Here's the drawing with two shaded views (mm, measured from the low corner). I have some questions. Coordinates: 2 decimals unless noted, no trailing zeros. Write each loop counter-clockwise with the first axis right and the second up, starting at its lowest first coordinate (ties: lowest second). Pieces come first, ordered by that corner, then holes.
Item 1: I want a section at B-B on z = 188.5. Please give me the cut outline in (x, y), then the cut area to 3 significant figures.
Item 2: For P1, Ø8, axis at x = 82.5, y = 184, coming from the -Z side, with a flat end and sliding along its axis, tell me the tip position at first contact or that it passes through.
Item 3: Thinking about a two-plate mould opening in Y: for the marked faces 1 and 2, which applies, +Y half, -Y half, draft (parallel to the pull), parting line (faces both ways), or undercut?
Item 4: I want a section at D-D on x = 172.5. Please give me the cut outline in (y, z).
Item 5: I want a section at A-A on y = 425. Please give me the cut outline in (x, z).
Item 6: If I drill on probe 1 along X at (y, z) = (24, 268); probe 2 along Z at (x, y) = (128, 170.5); probe 3 along X at (y, z) = (428.5, 295.5), over which ranges is the centre line in solid material (lowest first)?
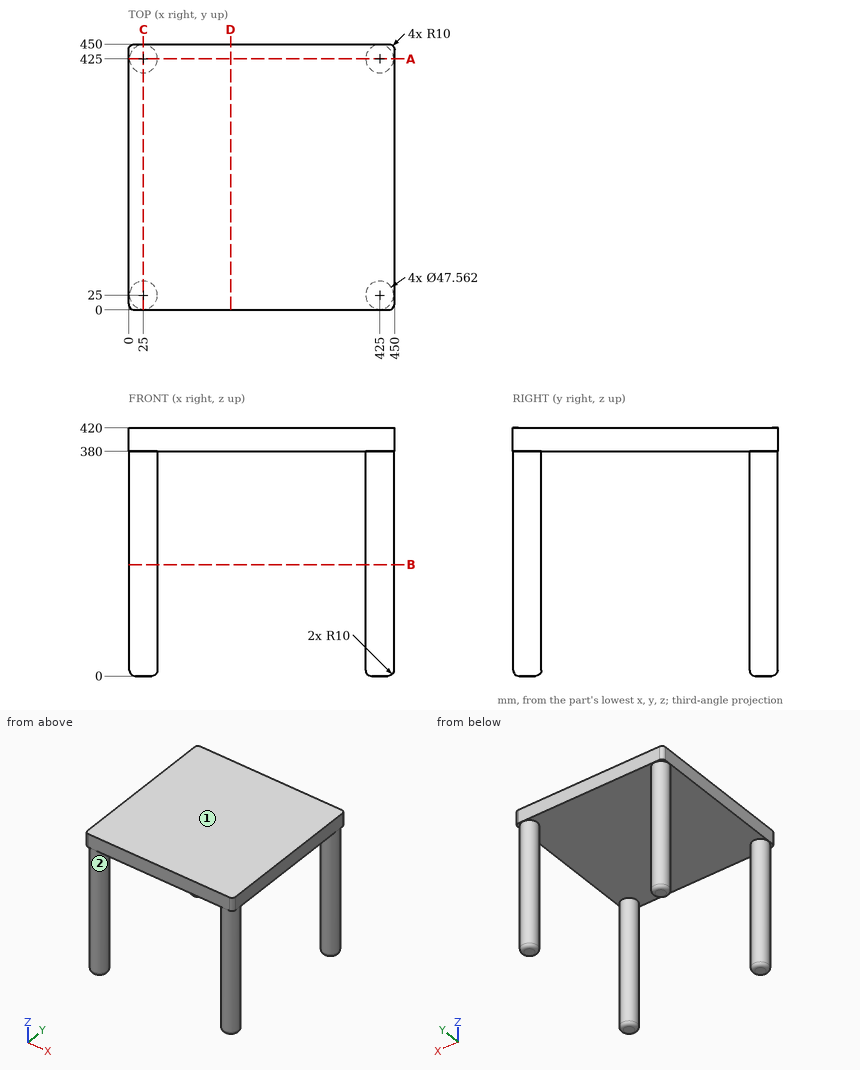
Response values:
1. outline: circle Ø47.56 at (25, 25); circle Ø47.56 at (25, 425); circle Ø47.56 at (425, 25); circle Ø47.56 at (425, 425)
1. area: 7,110 mm2
2. P1: stops at z = 380
3. face 1: draft
3. face 2: undercut
4. outline: (0, 380) - (450, 380) - (450, 420) - (0, 420) - close
5. outline: (0, 380) - (1.22, 380) - (1.22, 10) arc R10 ccw to (11.22, 0) - (38.78, 0) arc R10 ccw to (48.78, 10) - (48.78, 380) - (401.22, 380) - (401.22, 10) arc R10 ccw to (411.22, 0) - (438.78, 0) arc R10 ccw to (448.78, 10) - (448.78, 380) - (450, 380) - (450, 420) - (0, 420) - close
6. probe 1: x = 1.24 to 48.76, 401.24 to 448.76
6. probe 2: z = 380 to 420
6. probe 3: x = 1.48 to 48.52, 401.48 to 448.52
